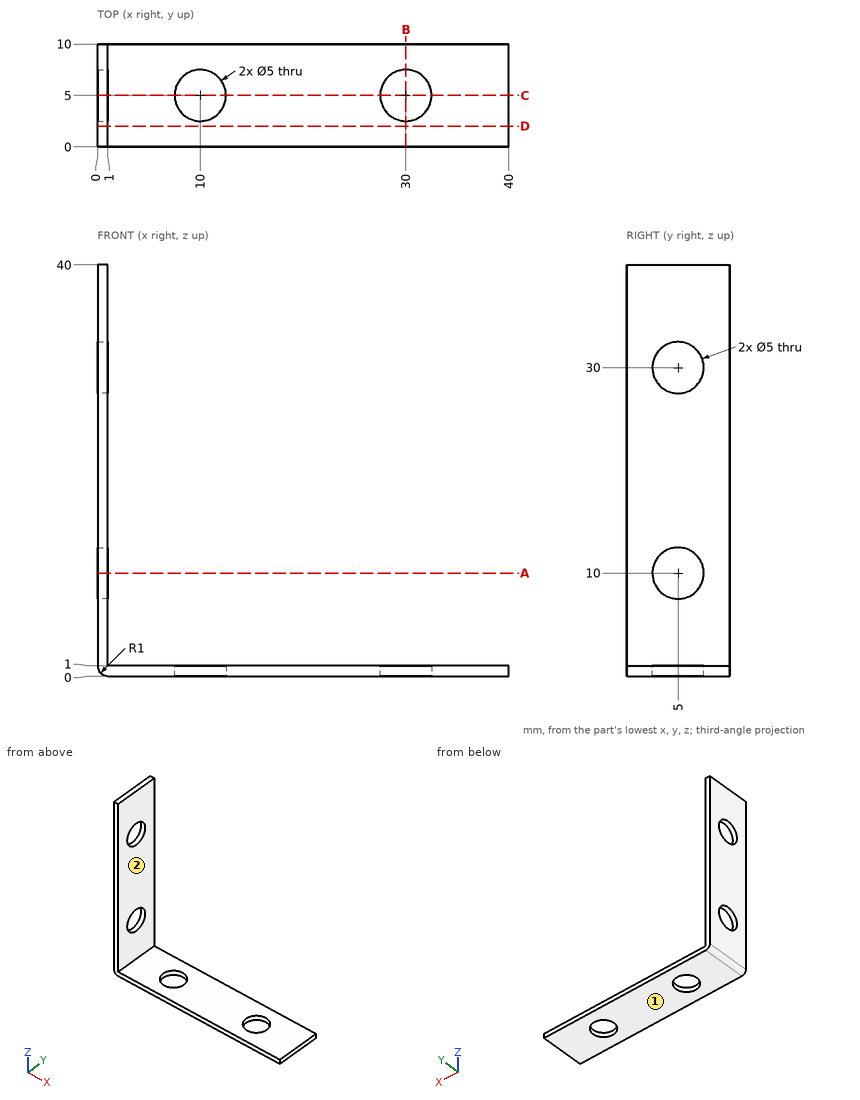
Check sheet for the drawn part. Datum: minimum x, y, z corner. Units: mm. A direction names the side the tool comes from. Round coordinates to 2 decimals unless told otherwise and drop trailing zeros. Order: outer loops, then holes, each group sorted by start corner. A loop starts at its lowest first (then second) coordinate and runs counter-clockwise, first axis right, second up.
1) Go/stop test with flat-tipped pins: pin 1 Ø4 at (y, z) = (5, 30) entering from +X; pin 2 Ø5 at (y, z) = (3, 22.5) entering from +X; pin 3 Ø4 at (x, y) = (11.5, 7) entering from +Z. Record where each tip stops, or that it passes through.
2) Section check B-B (x = 30). Record the boundary of the cut face in (y, z).
3) Section check A-A (z = 10). Record the boundary of the cut face in (x, y).
4) Section check C-C (y = 5). Record the boundary of the cut face in (x, z).
5) Scan lines: line 1 (Y direction, x = 10, z = 0.35); line 2 (X direction, y = 7.25, z = 24). Record each from-to range of solid material in increasing order.
6) Tool access check on the marked faces 1 and 2. Record the directions out of +Z, -Z, +X, -X, +Y, -Y that give a thin tool (end or side, any length) a straight path to the whole face; none if there is none.
7) Section check D-D (y = 2). Record the boundary of the cut face in (x, z).
Result:
1. pin 1: passes through
1. pin 2: stops at x = 1
1. pin 3: stops at z = 1
2. outline: (0, 0) - (2.5, 0) - (2.5, 1) - (0, 1) - close; (7.5, 0) - (10, 0) - (10, 1) - (7.5, 1) - close
3. outline: (0, 0) - (1, 0) - (1, 2.5) - (0, 2.5) - close; (0, 7.5) - (1, 7.5) - (1, 10) - (0, 10) - close
4. outline: (0, 1) arc R1 ccw to (1, 0) - (7.5, 0) - (7.5, 1) - (1, 1) - (1, 7.5) - (0, 7.5) - close; (0, 12.5) - (1, 12.5) - (1, 27.5) - (0, 27.5) - close; (0, 32.5) - (1, 32.5) - (1, 40) - (0, 40) - close; (12.5, 0) - (27.5, 0) - (27.5, 1) - (12.5, 1) - close; (32.5, 0) - (40, 0) - (40, 1) - (32.5, 1) - close
5. line 1: y = 0 to 2.5, 7.5 to 10
5. line 2: x = 0 to 1
6. face 1: -Z, +X, -X, +Y, -Y
6. face 2: +Z, +X, +Y, -Y
7. outline: (0, 1) arc R1 ccw to (1, 0) - (40, 0) - (40, 1) - (1, 1) - (1, 40) - (0, 40) - close
